from build123d import *
from build123d.topology import SkipClean

# Parameters (mm, degrees)
BOSS_EXTRUDE1_DEPTH      = 5
BOSS_EXTRUDE1_DEPTH_BACK = 5
SKETCH2_R                = 7.5
BOSS_EXTRUDE2_DEPTH      = 7.5
BOSS_EXTRUDE2_DEPTH_BACK = 7.5
BOSS_EXTRUDE3_DEPTH      = 7.5
BOSS_EXTRUDE3_DEPTH_BACK = 7.5
SKETCH5_R                = 12.5
SKETCH5_R_2              = 7.5
CUT_EXTRUDE1_DEPTH       = 1.5
FILLET1_R                = 10
TAP_DRILL_FOR_M6_TAP1_D  = 5


with BuildPart() as part:
    # Sketch2 → Boss-Extrude1 (new, two sides: drawn at the far end of the back side and taken through both)
    with BuildSketch(Plane.XY.offset(-BOSS_EXTRUDE1_DEPTH_BACK)):
        with BuildLine():
            Line((-27.5, 0), (-16, 0))
            ThreePointArc((-16, 0), (0, 16), (16, 0))
            Line((16, 0), (27.5, 0))
            Line((27.5, 0), (27.5, 15))
            Line((27.5, 15), (20, 15))
            ThreePointArc((20, 15), (12.565835097, 29.188611699), (10, 45))
            Line((10, 45), (10, 122.5))
            ThreePointArc((10, 122.5), (0, 142.5), (-10, 122.5))
            Line((-10, 122.5), (-10, 45))
            ThreePointArc((-10, 45), (-12.565835097, 29.188611699), (-20, 15))
            Line((-20, 15), (-27.5, 15))
            Line((-27.5, 15), (-27.5, 0))
        make_face()
        with Locations((0, 130)):
            Circle(SKETCH2_R, mode=Mode.SUBTRACT)
    extrude(amount=BOSS_EXTRUDE1_DEPTH + BOSS_EXTRUDE1_DEPTH_BACK)

    # Sketch3 → Boss-Extrude2 (add, two sides: drawn at the far end of the back side and taken through both)
    with BuildSketch(Plane.XY.offset(-BOSS_EXTRUDE2_DEPTH_BACK)):
        with BuildLine():
            Line((-27.5, 15), (-27.5, 0))
            Line((-27.5, 0), (-16, 0))
            ThreePointArc((-16, 0), (0, 16), (16, 0))
            Line((16, 0), (27.5, 0))
            Line((27.5, 0), (27.5, 15))
            Line((27.5, 15), (20, 15))
            ThreePointArc((20, 15), (0, 25), (-20, 15))
            Line((-20, 15), (-27.5, 15))
        make_face()
    extrude(amount=BOSS_EXTRUDE2_DEPTH + BOSS_EXTRUDE2_DEPTH_BACK)

    # Sketch5 → Boss-Extrude3 (add, two sides: drawn at the far end of the back side and taken through both)
    with SkipClean():  # the faces are left unmerged after this step: merging them gives an invalid solid
        with BuildSketch(Plane.XY.offset(-BOSS_EXTRUDE3_DEPTH_BACK)):
            with Locations((0, 130)):
                Circle(SKETCH5_R)
            with Locations((0, 130)):
                Circle(SKETCH5_R_2, mode=Mode.SUBTRACT)
        extrude(amount=BOSS_EXTRUDE3_DEPTH + BOSS_EXTRUDE3_DEPTH_BACK)
    add(part.part.scale(1), mode=Mode.REPLACE)  # the faces are merged on a copy

    # Sketch6 → Cut-Extrude1 (cut)
    with BuildSketch(Plane.XY.offset(5)):
        with BuildLine():
            Line((-6, 31.749015733), (-6, 113.477288358))
            ThreePointArc((-6, 113.477288358), (-5.236693885, 115.049098854), (-3.529411765, 115.421136787))
            ThreePointArc((-3.529411765, 115.421136787), (0, 115), (3.529411765, 115.421136787))
            ThreePointArc((3.529411765, 115.421136787), (5.236693885, 115.049098854), (6, 113.477288358))
            Line((6, 113.477288358), (6, 31.749015733))
            ThreePointArc((6, 31.749015733), (5.322875656, 30.249015733), (3.75, 29.764702249))
            ThreePointArc((3.75, 29.764702249), (0, 30), (-3.75, 29.764702249))
            ThreePointArc((-3.75, 29.764702249), (-5.322875656, 30.249015733), (-6, 31.749015733))
        make_face()
    cut_extrude1 = extrude(amount=-CUT_EXTRUDE1_DEPTH, mode=Mode.SUBTRACT)

    # Mirror1: Cut-Extrude1 across plane
    add(cut_extrude1.mirror(Plane.XY), mode=Mode.SUBTRACT)

    # Fillet1
    # the kernel refuses this fillet: 10 mm, written as the material it adds along each edge
    with BuildSketch(Plane(origin=(-10, 122.5, 5), x_dir=(0, -1, 0), z_dir=(0, 0, -1))) as fillet1_piece_1:
        with BuildLine():
            CenterArc((2.807764064, 10), FILLET1_R, 242.733955549, 27.266044451)
            ThreePointArc((-1.773464409, 1.111111111), (-0.863438171, 0.592735581), (0, 0))
            Line((0, 0), (2.807764064, 0))
        make_face()
    extrude(amount=10)
    with BuildSketch(Plane(origin=(10, 122.5, 5), x_dir=(0.5309249463264099, 0.8474188464792949, 0), z_dir=(0, 0, -1))) as fillet1_piece_2:
        with BuildLine():
            CenterArc((2.929897279, 9.96490045), FILLET1_R, 237.932028952, 27.266044451)
            Line((-2.379352184, 1.490711985), (0, 0))
            ThreePointArc((0, 0), (1.046391885, 0.043874438), (2.092783771, 0))
        make_face()
    extrude(amount=10)

    # Tap Drill for M6 Tap1 (through all)
    with Locations(Plane(origin=(0, 0, 0), x_dir=(-1, 0, 0), z_dir=(0, -1, 0))):
        with Locations((22, 0), (-22, 0)):
            Hole(TAP_DRILL_FOR_M6_TAP1_D / 2)


solid = part.part
The listing builds one solid part. Answer for the finished solid, in the listing's coordinates (mm). A direction names the side the tool comes from. Coordinates: 2 decimals unless noted, no trailing zeros. Write each loop counter-clockwise with the first axis right and the second up, starting at its lowest first coordinate (ties: lowest second). Pieces come first, ordered by that corner, then holes. Notation, with made-up numbers: (60, -36.5) - (75, -36.5) arc R23 ccw to (75, -10.5) - close; hole circle Ø8 at (-40, 5.5). An arc over 180 degrees is marked (long way). Put each result on its own line as item: value.
1. The part is cut by section D-D on x = 0. Give the vertices of the cut face in (y, z), plus the area to 3 significant figures.
Answer sheet:
outline: (16, -7.5) - (25, -7.5) - (25, -5) - (30, -5) - (30, -3.5) - (115, -3.5) - (115, -5) - (117.5, -5) - (117.5, -7.5) - (122.5, -7.5) - (122.5, 7.5) - (117.5, 7.5) - (117.5, 5) - (115, 5) - (115, 3.5) - (30, 3.5) - (30, 5) - (25, 5) - (25, 7.5) - (16, 7.5) - close; (137.5, -7.5) - (142.5, -7.5) - (142.5, 7.5) - (137.5, 7.5) - close
area: 955 mm^2
2. Find the intervals of material crossed by line 1 along Z through (x, y) = (-22, 3); line 2 along Y through (x, z) = (0, -4.25); line 3 along Y through (x, z) = (20, 5.5), in increasing order. Write a range as from..to.
Answer sheet:
line 1: z = -7.5..-2.5, 2.5..7.5
line 2: y = 16..30, 115..122.5, 137.5..142.5
line 3: y = 0..15
3. The part is cut by section A-A on x = -22. Give the vertices of the cut face in (y, z), plus the area to 3 significant figures.
Answer sheet:
outline: (0, -7.5) - (15, -7.5) - (15, -2.5) - (0, -2.5) - close; (0, 2.5) - (15, 2.5) - (15, 7.5) - (0, 7.5) - close
area: 150 mm^2
4. The part is cut by section B-B on z = 0. Give the vertices of the cut face in (x, y).
Answer sheet:
outline: (-27.5, 0) - (-24.5, 0) - (-24.5, 15) - (-27.5, 15) - close; (-19.5, 0) - (-16, 0) arc R16 cw to (16, 0) - (19.5, 0) - (19.5, 15.68) arc R50 cw to (10, 45) - (10, 119.69) arc R10 cw to (11.11, 124.27) arc R12.5 ccw (long way) to (-11.11, 124.27) arc R10 cw to (-10, 119.69) - (-10, 45) arc R50 cw to (-19.5, 15.68) - close; (24.5, 0) - (27.5, 0) - (27.5, 15) - (24.5, 15) - close; hole circle Ø15 at (0, 130)
5. Determine the mould class of faces 1 (the face through (-24.5, 7.9, -0.1)), 2 (the face through (-12.495, 29.402, -0.07)), 3 (the face through (0, 122, 7.5)) for opening direction X: pulls with the +X half, pulls with the -X half, needs draft (parallel to the pull), parting line crosses it, or undercut.
Answer sheet:
face 1: undercut
face 2: pulls with the -X half
face 3: needs draft
6. A tool of negligible diameter and unlimited length cuts with its end or side. For faces 4 (the face through (10, 82, 0)), 5 (the face through (0, 73, 3.5)), 6 (the face through (-10.29, 122.08, 0.07)), 7 (the face through (0, 25, -6)), 8 (the face through (-25, 15, 0)), from which of +Z, -Z, +X, -X, +Y, -Y can it reach the whole face along a straight path? Write none if from no direction.
Answer sheet:
face 4: +Z, -Z, +X
face 5: +Z
face 6: +Z, -Z, -X
face 7: -Z
face 8: +Z, -Z, -X, +Y
7. Flat-ended cylindrical pins translate along their axes: pin 1 Ø9.5 at (x, y) = (2.5, 82) entering from -Z; pin 2 Ø1.2 at (y, z) = (57.5, -4.5) entering from +X; pin 3 Ø6 at (x, z) = (-4, -1) entering from +Y. Find the tip coordinate at first contact, or state that the pin passes through.
Answer sheet:
pin 1: stops at z = -5
pin 2: stops at x = 10
pin 3: stops at y = 142.46
8. The part is cut by section C-C on y = 108. Give the vertices of the cut face in (x, z), plus the area to 3 significant figures.
Answer sheet:
outline: (-10, -5) - (-6, -5) - (-6, -3.5) - (6, -3.5) - (6, -5) - (10, -5) - (10, 5) - (6, 5) - (6, 3.5) - (-6, 3.5) - (-6, 5) - (-10, 5) - close
area: 164 mm^2
